Read the model definition and answer for the solid it produces. Units are mm, in the model's axes. A direction names the side the tool comes from. Coordinates: 2 decimals unless noted, no trailing zeros. Order: outer loops, then holes, each group sorted by start corner. A loop starts at its lowest first (then second) coordinate and runs counter-clockwise, first axis right, second up. Notation, with made-up numbers: M 31,27.25 L 44,27.25 A24 ccw 44,52.25 Z; hole C -12.75,46 d4. An arc over 180 degrees is marked long. One line per question, with ' | ' between items. Start each with the question number.
1) Consider probe 1 along Y at (x, z) = (-47, 2.45); probe 2 along X at (y, z) = (14, 2.2); probe 3 along X at (y, z) = (-10, 0.9). Determine where each line is inside the solid, lowest interval first.
2) A tool of negligible diameter and unlimited length cuts with its end or side. For faces 1 (the face through (-47.8, -15.4, 1.6)), 2 (the face through (-55.424, -14.666, 1.565)), 3 (the face through (-22.94, 44.76, 1.57)), from which of +Z, -Z, +X, -X, +Y, -Y can it reach the whole face along a straight path? Write none if from no direction.
3) Find section A-A, the plane y = 0. Write down the section's boundary in (x, z) (3 decimals).
4) The mould has two halves that part along X. Classify faces 4 (the face through (-38.91, 16.02, 1.57)), 5 (the face through (55.44, -14.6, 1.57)), 6 (the face through (12, 1, 0)): +X half, -X half, draft (parallel to the pull), parting line (faces both ways), or undercut.
5) Find section D-D, the plane x = 33. Write down the section's boundary in (y, z) (3 decimals).
6) Find section C-C, the plane z = 2.15. Count the separate pieces of the cut face and the enclosed holes in it, plus the area to 3 significant figures.
from build123d import *

# Parameters (mm, degrees)
SKETCH1_R           = 57.332002373
BOSS_EXTRUDE1_DEPTH = 3.175
CUT_EXTRUDE1_START  = -3.175
CUT_EXTRUDE1_DEPTH  = 3.175
CIRPATTERN1_COUNT   = 8
CUT_EXTRUDE2_REACH  = 81.25
SKETCH3_R           = 3.175
CUT_EXTRUDE3_REACH  = 81.25
SKETCH4_R           = 0.762
CHAMFER1_SIZE       = 3.175
CUT_EXTRUDE4_REACH  = 81.25
SKETCH5_R           = 1.4986
CIRPATTERN2_COUNT   = 4


with BuildPart() as part:
    # Sketch1 → Boss-Extrude1 (new body)
    with BuildSketch(Plane.XY):
        Circle(SKETCH1_R)
    extrude(amount=BOSS_EXTRUDE1_DEPTH)

    # Sketch2 → Cut-Extrude1 (cut)
    with BuildSketch(Plane.XY.offset(3.175).offset(CUT_EXTRUDE1_START)):
        with BuildLine():
            Line((62.131865528, 30.134703259), (41.073015989, 21.411842172))
            ThreePointArc((41.073015989, 21.411842172), (38.873595038, 16.101970283), (44.183466927, 13.902549332))
            Line((44.183466927, 13.902549332), (54.389846688, 18.130170251))
            ThreePointArc((54.389846688, 18.130170251), (55.267949497, 15.245073122), (55.99312865, 12.317793637))
            ThreePointArc((55.99312865, 12.317793637), (52.309071806, 0), (55.99312865, -12.317793637))
            ThreePointArc((55.99312865, -12.317793637), (55.267949497, -15.245073122), (54.389846688, -18.130170251))
            Line((54.389846688, -18.130170251), (44.183466927, -13.902549332))
            ThreePointArc((44.183466927, -13.902549332), (38.873595038, -16.101970283), (41.073015989, -21.411842172))
            Line((41.073015989, -21.411842172), (62.131865528, -30.134703259))
            ThreePointArc((62.131865528, -30.134703259), (69.054102373, 0), (62.131865528, 30.134703259))
        make_face()
    cut_extrude1 = extrude(amount=CUT_EXTRUDE1_DEPTH, mode=Mode.SUBTRACT)

    # CirPattern1: Cut-Extrude1 ×8 about axis
    cirpattern1_axis = Axis((0, 0, 0), (0, 0, 1))
    for i in range(1, CIRPATTERN1_COUNT):
        add(cut_extrude1.rotate(cirpattern1_axis, i * 360 / CIRPATTERN1_COUNT), mode=Mode.SUBTRACT)

    # Sketch3 → Cut-Extrude2 (cut, up to next)
    with BuildSketch(Plane.XY.offset(3.175), mode=Mode.PRIVATE) as cut_extrude2_sk1:
        Circle(SKETCH3_R)
    cut_extrude2_tool1 = extrude(cut_extrude2_sk1.sketch, amount=-CUT_EXTRUDE2_REACH, mode=Mode.PRIVATE) & part.part
    add(cut_extrude2_tool1.solids().sort_by_distance((0, 0, 3.175))[0], mode=Mode.SUBTRACT)

    # Sketch4 → Cut-Extrude3 (cut, up to next)
    with BuildSketch(Plane.XY.offset(3.175), mode=Mode.PRIVATE) as cut_extrude3_sk1:
        with Locations((6.873190472, 16.593349654)):
            Circle(SKETCH4_R)
    cut_extrude3_tool1 = extrude(cut_extrude3_sk1.sketch, amount=-CUT_EXTRUDE3_REACH, mode=Mode.PRIVATE) & part.part
    # Sketch4 → Cut-Extrude3 (cut, up to next)
    with BuildSketch(Plane.XY.offset(3.175), mode=Mode.PRIVATE) as cut_extrude3_sk2:
        with Locations((-6.873190472, -16.593349654)):
            Circle(SKETCH4_R)
    cut_extrude3_tool2 = extrude(cut_extrude3_sk2.sketch, amount=-CUT_EXTRUDE3_REACH, mode=Mode.PRIVATE) & part.part
    add(cut_extrude3_tool1.solids().sort_by_distance((6.87319, 16.59335, 3.175))[0], mode=Mode.SUBTRACT)
    add(cut_extrude3_tool2.solids().sort_by_distance((-6.87319, -16.59335, 3.175))[0], mode=Mode.SUBTRACT)

    # Chamfer1
    # the kernel refuses this chamfer: 3.175, 1.27 mm, written as the material it takes off along each edge
    with BuildSketch(Plane(origin=(-51.279395749, 25.639463092, -8.232085276), x_dir=(0.4570542890286377, 0.8894387988392043, 0), z_dir=(0, 0, 1)), Plane(origin=(-18.130170251, 54.389846688, -8.232085276), x_dir=(0.9521143932521638, 0.3057420189670758, 0), z_dir=(0, 0, 1)), Plane(origin=(25.639463092, 51.279395749, -8.232085276), x_dir=(0.8894387988392037, -0.4570542890286388, 0), z_dir=(0, 0, 1)), Plane(origin=(54.389846688, 18.130170251, -8.232085276), x_dir=(0.30574201896707504, -0.9521143932521642, 0), z_dir=(0, 0, 1)), Plane(origin=(25.639463092, -51.279395749, 11.407085276), x_dir=(0.8894387988391999, 0.45705428902864664, 0), z_dir=(0, 0, -1)), Plane(origin=(-18.130170251, -54.389846688, 11.407085276), x_dir=(0.952114393252168, -0.305742018967063, 0), z_dir=(0, 0, -1)), Plane(origin=(-51.279395749, -25.639463092, 11.407085276), x_dir=(0.4570542890286467, -0.8894387988391996, 0), z_dir=(0, 0, -1))) as chamfer1_piece_1:
        with BuildLine():
            Line((1.265469022, 0), (CHAMFER1_SIZE * 0.0818896104616, -CHAMFER1_SIZE * 0.996641405772))
            Line((CHAMFER1_SIZE * 0.0818896104616, -CHAMFER1_SIZE * 0.996641405772), (0, 0))
            ThreePointArc((0, 0), (0.65194513, 0.003488419), (1.265469022, 0))
        make_face()
    extrude(amount=19.639170553, mode=Mode.SUBTRACT)
    with BuildSketch(Plane(origin=(-54.389846688, 18.130170251, 11.407085276), x_dir=(0.9238795325112874, -0.3826834323650885, 0), z_dir=(0, 0, -1)), Plane(origin=(-25.639463092, 51.279395749, 11.407085276), x_dir=(0.3826834323650902, -0.9238795325112866, 0), z_dir=(0, 0, -1)), Plane(origin=(18.130170251, 54.389846688, 11.407085276), x_dir=(-0.3826834323650892, -0.923879532511287, 0), z_dir=(0, 0, -1)), Plane(origin=(51.279395749, 25.639463092, 11.407085276), x_dir=(-0.9238795325112859, -0.38268343236509195, 0), z_dir=(0, 0, -1)), Plane(origin=(18.130170251, -54.389846688, -8.232085276), x_dir=(-0.38268343236509117, 0.9238795325112862, 0), z_dir=(0, 0, 1)), Plane(origin=(-25.639463092, -51.279395749, -8.232085276), x_dir=(0.3826834323650892, 0.923879532511287, 0), z_dir=(0, 0, 1)), Plane(origin=(-54.389846688, -18.130170251, -8.232085276), x_dir=(0.9238795325112866, 0.3826834323650902, 0), z_dir=(0, 0, 1))) as chamfer1_piece_2:
        with BuildLine():
            Line((CHAMFER1_SIZE, 0), (0.103628765, 1.261218825))
            ThreePointArc((0.103628765, 1.261218825), (0.04991083, 0.650041176), (0, 0))
            Line((0, 0), (CHAMFER1_SIZE, 0))
        make_face()
    extrude(amount=19.639170553, mode=Mode.SUBTRACT)
    with BuildSketch(Plane(origin=(51.279395749, -25.639463092, 11.407085276), x_dir=(-0.9238795325112863, 0.382683432365091, 0), z_dir=(0, 0, -1))) as chamfer1_piece_3:
        with BuildLine():
            Line((CHAMFER1_SIZE, 0), (0.103628765, -1.261218825))
            ThreePointArc((0.103628765, -1.261218825), (0.04991083, -0.650041176), (0, 0))
            Line((0, 0), (CHAMFER1_SIZE, 0))
        make_face()
    extrude(amount=19.639170553, mode=Mode.SUBTRACT)
    with BuildSketch(Plane(origin=(54.389846688, -18.130170251, -8.232085276), x_dir=(0.3057420189670742, 0.9521143932521645, 0), z_dir=(0, 0, 1))) as chamfer1_piece_4:
        with BuildLine():
            Line((1.265469022, 0), (CHAMFER1_SIZE * 0.0818896104616, CHAMFER1_SIZE * 0.996641405772))
            Line((CHAMFER1_SIZE * 0.0818896104616, CHAMFER1_SIZE * 0.996641405772), (0, 0))
            ThreePointArc((0, 0), (0.65194513, -0.003488419), (1.265469022, 0))
        make_face()
    extrude(amount=19.639170553, mode=Mode.SUBTRACT)

    # Sketch5 → Cut-Extrude4 (cut, up to next)
    with BuildSketch(Plane.XY.offset(3.175), mode=Mode.PRIVATE) as cut_extrude4_sk1:
        with Locations((-10.93517908, 26.399857642)):
            Circle(SKETCH5_R)
    cut_extrude4_tool1 = extrude(cut_extrude4_sk1.sketch, amount=-CUT_EXTRUDE4_REACH, mode=Mode.PRIVATE) & part.part
    cut_extrude4 = cut_extrude4_tool1.solids().sort_by_distance((-10.935179, 26.399858, 3.175))[0]
    add(cut_extrude4, mode=Mode.SUBTRACT)

    # CirPattern2: Cut-Extrude4 ×4 about axis
    cirpattern2_axis = Axis((0, 0, 0), (0, 0, 1))
    for i in range(1, CIRPATTERN2_COUNT):
        add(cut_extrude4.rotate(cirpattern2_axis, i * 360 / CIRPATTERN2_COUNT), mode=Mode.SUBTRACT)


solid = part.part
Report:
1) probe 1: y = -31.19 to -23.87, -15.07 to 15.07, 23.87 to 31.19 | probe 2: x = -55.6 to -44.42, -40.86 to 40.86, 44.42 to 55.6 | probe 3: x = -54.66 to -27.57, -25.23 to 54.66
2) face 1: +Z, -Z | face 2: +Z, -Z, -X, -Y | face 3: +Z, -Z, +Y
3) outline: M -52.309,0 L -3.175,0 L -3.175,3.175 L -52.309,3.175 Z; M 3.175,0 L 52.309,0 L 52.309,3.175 L 3.175,3.175 Z
4) face 4: undercut | face 5: +X half | face 6: draft
5) outline: M -42.401,0 L 42.401,0 L 42.401,3.175 L -42.401,3.175 Z
6) separate pieces: 1 | enclosed holes: 7 | area: 8,630 mm^2
